Check sheet for the drawn part. Datum: minimum x, y, z corner. Units: mm. A direction names the side the tool comes from. Round coordinates to 2 decimals unless told otherwise and drop trailing zeros. Order: outer loops, then holes, each group sorted by start corner. A loop starts at its lowest first (then second) coordinate and runs counter-clockwise, first axis right, second up.
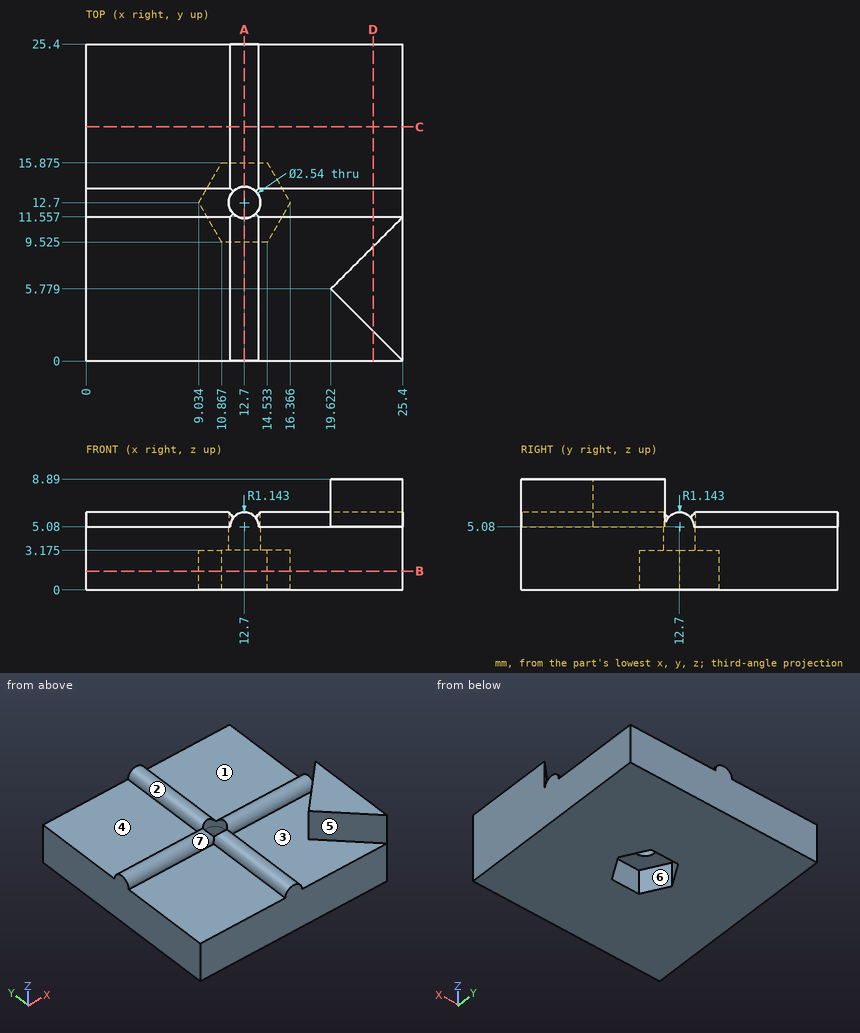
1) Scan lines: line 1 (Y direction, x = 12.7, z = 4.4); line 2 (Y direction, x = 13.75, z = 1) (1 decimal); line 3 (Z direction, x = 3.5, y = 20.5). Record each from-to range of solid material in increasing order.
2) Sectioned sample at D-D on x = 23. Record the cut outline in (y, z) (1 decimal).
3) Sectioned sample at B-B on z = 1.5. Record the cut outline in (x, y) (1 decimal).
4) Sectioned sample at C-C on y = 18.75. Record the cut outline in (x, z) (1 decimal), and give its area (3 significant figures).
5) Set-up check for the marked faces 1, 2, 3 and 4: record each of +Z, -Z, +X, -X, +Y, -Y from which the full face is reachable in a straight line by a thin tool's end or side.
6) Sectioned sample at A-A on x = 12.7. Record the cut outline in (y, z) (1 decimal).
7) Draft check along Y on the marked faces 5, 6 and 7. Enter one of: pulls with the +Y half, pulls with the -Y half, needs draft (parallel to the pull), parting line crosses it, or undercut.
8) Gauge pin test, flat ends, axial feed: pin 1 (2 mm diameter, centred on x = 11.5, y = 22.5, fed in from +Z) (1 decimal); pin 2 (6 mm diameter, centred on x = 3.5, y = 20.5, fed in from +Z); pin 3 (1 mm diameter, centred on y = 12, z = 7.5, fed in from -X) (1 decimal). Record the tip position at first contact, or that the pin passes through.
Values found:
1. line 1: y = 0 to 11.43, 13.97 to 25.4
1. line 2: y = 0 to 9.5, 15.9 to 25.4
1. line 3: z = 0 to 5.08
2. outline: (0, 0) - (25.4, 0) - (25.4, 5.1) - (13.8, 5.1) arc R1.1 ccw to (11.6, 5.1) - (9.2, 5.1) - (9.2, 8.9) - (2.4, 8.9) - (2.4, 5.1) - (0, 5.1) - close
3. outline: (0, 0) - (25.4, 0) - (25.4, 25.4) - (0, 25.4) - close; hole (9, 12.7) - (10.9, 9.5) - (14.5, 9.5) - (16.4, 12.7) - (14.5, 15.9) - (10.9, 15.9) - close
4. outline: (0, 0) - (25.4, 0) - (25.4, 5.1) - (13.8, 5.1) arc R1.1 ccw to (11.6, 5.1) - (0, 5.1) - close
4. area: 131 mm2
5. face 1: +Z, +X, +Y
5. face 2: +Z, +Y
5. face 3: +Z
5. face 4: +Z, -X, +Y
6. outline: (0, 0) - (9.5, 0) - (9.5, 3.2) - (11.4, 3.2) - (11.4, 6.2) - (0, 6.2) - close; (14, 3.2) - (15.9, 3.2) - (15.9, 0) - (25.4, 0) - (25.4, 6.2) - (14, 6.2) - close
7. face 5: pulls with the -Y half
7. face 6: undercut
7. face 7: parting line crosses it
8. pin 1: stops at z = 6.2
8. pin 2: stops at z = 5.08
8. pin 3: stops at x = 25.3
